Autodesk Inventor part; units mm, degrees
ref_plane "YZ Plane" through (0, 0, 0) normal (1, 0, 0) x (0, 1, 0)
ref_plane "XZ Plane" through (0, 0, 0) normal (0, 1, 0) x (-1, 0, 0)
ref_plane "XY Plane" through (0, 0, 0) normal (0, 0, 1) x (1, 0, 0)
sketch "Sketch1" plane through (0, 0, 0) normal (1, 0, 0) x (0, 1, 0)
  line L0 (-1.5875, -355.6) -> (1.5875, -355.6) construction
  line L1 (1.5875, -355.6) -> (1.5875, 355.6) construction
  line L2 (1.5875, 355.6) -> (-1.5875, 355.6) construction
  line L3 (-1.5875, 355.6) -> (-1.5875, -355.6) construction
  line L4 (-1.5875, -355.6) -> (1.5875, 355.6) construction
  line L5 (1.5875, -355.6) -> (-1.5875, 355.6) construction
  line L6 (52.3875, 152.4) -> (1.5875, 152.4) construction
  line L7 (1.5875, 152.4) -> (1.5875, 127) construction
  line L8 (1.5875, 127) -> (52.3875, 127) construction
  line L9 (52.3875, 127) -> (52.3875, 152.4) construction
  line L10 (52.3875, 152.4) -> (1.5875, 127) construction
  line L11 (1.5875, 152.4) -> (52.3875, 127) construction
  line L12 (77.7875, 177.8) -> (1.5875, 177.8) construction
  line L13 (1.5875, 177.8) -> (1.5875, 152.4) construction
  line L14 (1.5875, 152.4) -> (77.7875, 152.4) construction
  line L15 (77.7875, 152.4) -> (77.7875, 177.8) construction
  line L16 (77.7875, 177.8) -> (1.5875, 152.4) construction
  line L17 (1.5875, 177.8) -> (77.7875, 152.4) construction
  line L18 (900.1125, 152.4) -> (87.3125, 152.4) construction
  line L19 (87.3125, 152.4) -> (87.3125, 177.8) construction
  line L20 (87.3125, 177.8) -> (900.1125, 177.8) construction
  line L21 (900.1125, 177.8) -> (900.1125, 152.4) construction
  line L22 (900.1125, 152.4) -> (87.3125, 177.8) construction
  line L23 (87.3125, 152.4) -> (900.1125, 177.8) construction
  line L24 (87.3125, 177.8) -> (77.7875, 177.8) construction
  line L25 (77.7875, 177.8) -> (77.7875, -177.8) construction
  line L26 (77.7875, -177.8) -> (87.3125, -177.8) construction
  line L27 (87.3125, -177.8) -> (87.3125, 177.8) construction
  line L28 (87.3125, 177.8) -> (77.7875, -177.8) construction
  line L29 (77.7875, 177.8) -> (87.3125, -177.8) construction
  line L30 (82.55, 0) -> (-1.5875, 0) construction
  line L31 (1.5875, -355.6) -> (-1.5875, -355.6) construction
  line L32 (52.3875, -152.4) -> (1.5875, -152.4) construction
  line L33 (1.5875, -152.4) -> (1.5875, -127) construction
  line L34 (1.5875, -127) -> (52.3875, -127) construction
  line L35 (52.3875, -127) -> (52.3875, -152.4) construction
  line L36 (52.3875, -152.4) -> (1.5875, -127) construction
  line L37 (1.5875, -152.4) -> (52.3875, -127) construction
  line L38 (77.7875, -177.8) -> (1.5875, -177.8) construction
  line L39 (1.5875, -177.8) -> (1.5875, -152.4) construction
  line L40 (1.5875, -152.4) -> (77.7875, -152.4) construction
  line L41 (77.7875, -152.4) -> (77.7875, -177.8) construction
  line L42 (77.7875, -177.8) -> (1.5875, -152.4) construction
  line L43 (1.5875, -177.8) -> (77.7875, -152.4) construction
  line L44 (900.1125, -152.4) -> (87.3125, -152.4) construction
  line L45 (87.3125, -152.4) -> (87.3125, -177.8) construction
  line L46 (87.3125, -177.8) -> (900.1125, -177.8) construction
  line L47 (900.1125, -177.8) -> (900.1125, -152.4) construction
  line L48 (900.1125, -152.4) -> (87.3125, -177.8) construction
  line L49 (87.3125, -152.4) -> (900.1125, -177.8) construction
  line L50 (87.3125, -177.8) -> (77.7875, -177.8) construction
  circle A0 centre (66.6623, 160.02) radius 10.3124 construction
  circle A1 centre (66.6623, -160.02) radius 10.3124 construction
  line L51 (138.1125, 176.2125) -> (138.1125, 109.4105) construction
  line L52 (138.1125, 109.4105) -> (-27.5223, 109.4105) construction
  point P0 (0, 0)
  point P1 (26.9875, 139.7)
  point P2 (39.6875, 165.1)
  point P3 (1.5875, 165.1)
  point P4 (493.7125, 165.1)
  point P5 (26.9875, -139.7)
  point P6 (39.6875, -165.1)
  point P7 (1.5875, -165.1)
  point P8 (493.7125, -165.1)
  dimension "d0" = 3.175
  dimension "d1" = 711.2
  dimension "d2" = 50.8
  dimension "d3" = 25.4
  dimension "d4" = 139.7
  dimension "d5" = 76.2
  dimension "d6" = 25.4
  dimension "d7" = 812.8
  dimension "d8" = 25.4
  dimension "d9" = 9.525
  dimension "d10" = 355.6
  dimension "d11" = 20.6248
  dimension "d12" = 11.1252
  dimension "d13" = 7.62
  dimension "d23" = 66.802
  dimension "d24" = 50.8
sketch "Sketch3" plane through (0, 0, 0) normal (1, 0, 0) x (0, 1, 0)
  line L0 (77.7875, -152.4) -> (77.7875, -177.8) construction
  circle A0 centre (66.6623, -160.02) radius 10.3124 construction
  line L1 (1.5875, 355.6) -> (-1.5875, 355.6) construction
  line L2 (1.5875, -355.6) -> (1.5875, 355.6) construction
  line L3 (-1.5875, -355.6) -> (1.5875, 355.6) construction
  line L4 (1.5875, -355.6) -> (-1.5875, 355.6) construction
  line L5 (-1.5875, 355.6) -> (-1.5875, -355.6) construction
  line L6 (87.3125, -177.8) -> (87.3125, 177.8) construction
  line L7 (77.7875, 177.8) -> (77.7875, -177.8) construction
  line L8 (-1.5875, -355.6) -> (1.5875, -355.6) construction
  line L9 (1.5875, -355.6) -> (-1.5875, -355.6) construction
  line L10 (1.5875, 152.4) -> (1.5875, 127) construction
  line L11 (82.55, 0) -> (-1.5875, 0) construction
  line L12 (87.3125, 152.4) -> (87.3125, 177.8) construction
  line L13 (77.7875, -177.8) -> (87.3125, -177.8) construction
  line L14 (1.5875, -127) -> (52.3875, -127) construction
  line L15 (52.3875, 152.4) -> (1.5875, 152.4) construction
  line L16 (52.3875, 152.4) -> (1.5875, 127) construction
  line L17 (1.5875, 127) -> (52.3875, 127) construction
  line L18 (52.3875, 127) -> (52.3875, 152.4) construction
  line L19 (1.5875, 152.4) -> (52.3875, 127) construction
  line L20 (1.5875, 152.4) -> (77.7875, 152.4) construction
  line L21 (1.5875, 177.8) -> (1.5875, 152.4) construction
  line L22 (138.1125, 109.4105) -> (-27.5223, 109.4105) construction
  circle A1 centre (66.6623, 160.02) radius 10.3124 construction
  line L23 (138.1125, 176.2125) -> (138.1125, 109.4105) construction
  line L24 (77.7875, 177.8) -> (1.5875, 152.4) construction
  line L25 (77.7875, 177.8) -> (1.5875, 177.8) construction
  line L26 (77.7875, 152.4) -> (77.7875, 177.8) construction
  line L27 (87.3125, 177.8) -> (77.7875, 177.8) construction
  line L28 (1.5875, 177.8) -> (77.7875, 152.4) construction
  line L29 (900.1125, 152.4) -> (87.3125, 152.4) construction
  line L30 (87.3125, 177.8) -> (900.1125, 177.8) construction
  line L31 (900.1125, 152.4) -> (87.3125, 177.8) construction
  line L32 (87.3125, 152.4) -> (900.1125, 177.8) construction
  line L33 (900.1125, -152.4) -> (87.3125, -177.8) construction
  line L34 (87.3125, -177.8) -> (900.1125, -177.8) construction
  line L35 (900.1125, -152.4) -> (87.3125, -152.4) construction
  line L36 (87.3125, -152.4) -> (900.1125, -177.8) construction
  line L37 (900.1125, 177.8) -> (900.1125, 152.4) construction
  line L38 (900.1125, -177.8) -> (900.1125, -152.4) construction
  line L39 (52.3875, -127) -> (52.3875, -152.4) construction
  line L40 (52.3875, -152.4) -> (1.5875, -127) construction
  line L41 (1.5875, -152.4) -> (1.5875, -127) construction
  line L42 (1.5875, -152.4) -> (52.3875, -127) construction
  line L43 (52.3875, -152.4) -> (1.5875, -152.4) construction
  line L44 (1.5875, -152.4) -> (77.7875, -152.4) construction
  line L45 (1.5875, -177.8) -> (77.7875, -152.4) construction
  line L46 (77.7875, -177.8) -> (1.5875, -177.8) construction
  line L47 (1.5875, -177.8) -> (1.5875, -152.4) construction
  line L48 (77.7875, -177.8) -> (1.5875, -152.4) construction
  line L49 (87.3125, -152.4) -> (87.3125, -177.8) construction
  line L50 (87.3125, -177.8) -> (77.7875, -177.8) construction
  circle A2 centre (39.6875, 64.1731) radius 28.6512 construction
  circle A3 centre (65.0875, 99.0981) radius 10.3124 construction
  line L51 (57.4199, 164.5943) -> (14.0091, 76.8819) construction
  circle A4 centre (39.6875, 64.1731) radius 25.4 construction
  circle A5 centre (49.2125, 27.2829) radius 12.7 construction
  circle A6 centre (49.2125, 27.2829) radius 25.4 construction
  circle A7 centre (39.6875, -3.0046) radius 6.35 construction
  circle A8 centre (39.6875, -3.0046) radius 25.4 construction
  circle A9 centre (39.6875, -3.0046) radius 30.48 construction
  circle A10 centre (65.0875, 99.0981) radius 4.7625 construction
  circle A11 centre (39.6875, 64.1731) radius 14.2875
  circle A12 centre (49.2125, 27.2829) radius 14.2875
  circle A13 centre (9.2075, 45.1231) radius 4.7625 construction
  circle A14 centre (9.2075, 19.7231) radius 4.7625 construction
  line L52 (87.3125, 0) -> (87.3125, 86.6661)
  line L53 (87.3125, 86.6661) -> (68.1488, 102.7464)
  circle A15 centre (42.8625, 99.0981) radius 4.7625 construction
  line L54 (65.0875, 103.8606) -> (42.8625, 103.8606)
  line L55 (38.8212, 101.6179) -> (5.1662, 47.6429)
  line L56 (4.445, 45.1231) -> (4.445, 0)
  arc A16 (68.1488, 102.7464) -> (65.0875, 103.8606) centre (65.0875, 99.0981) ccw
  arc A17 (42.8625, 103.8606) -> (38.8212, 101.6179) centre (42.8625, 99.0981) ccw
  arc A18 (5.1662, 47.6429) -> (4.445, 45.1231) centre (9.2075, 45.1231) ccw
  line L57 (87.3125, 0) -> (87.3125, -86.6661)
  line L58 (87.3125, -86.6661) -> (68.1488, -102.7464)
  line L59 (65.0875, -103.8606) -> (42.8625, -103.8606)
  line L60 (38.8212, -101.6179) -> (5.1662, -47.6429)
  line L61 (4.445, -45.1231) -> (4.445, 0)
  arc A19 (65.0875, -103.8606) -> (68.1488, -102.7464) centre (65.0875, -99.0981) ccw
  arc A20 (38.8212, -101.6179) -> (42.8625, -103.8606) centre (42.8625, -99.0981) ccw
  arc A21 (4.445, -45.1231) -> (5.1662, -47.6429) centre (9.2075, -45.1231) ccw
  circle A22 centre (39.6875, -3.0046) radius 7.62
  circle A23 centre (39.6875, -64.1731) radius 14.2875
  circle A24 centre (49.2125, -27.2829) radius 14.2875
  point P0 (0, 0)
  point P1 (0, 0)
  point P2 (26.9875, 139.7)
  point P3 (1.5875, 165.1)
  point P4 (39.6875, 165.1)
  point P5 (493.7125, -165.1)
  point P6 (493.7125, 165.1)
  point P7 (26.9875, -139.7)
  point P8 (1.5875, -165.1)
  point P9 (39.6875, -165.1)
  point P10 (65.0875, -3.0046)
  point P11 (52.3875, 18.9924)
  point P12 (26.9875, 18.9924)
  point P13 (14.2875, -3.0046)
  point P14 (26.9875, -25.0017)
  point P15 (52.3875, -25.0017)
  point P16 (82.55, 76.2)
  point P17 (82.55, 25.4)
  point P18 (82.55, 177.8)
  dimension "d30" = 57.3024
  dimension "d36" = 50.8
  dimension "d31" = 12.7
  dimension "d32" = 50.8
  dimension "d33" = 25.4
  dimension "d34" = 50.8
  dimension "d35" = 12.7
  dimension "d37" = 60.96
  dimension "d38" = 38.1
  dimension "d39" = 34.925
  dimension "d40" = 9.525
  dimension "d41" = 28.575
  dimension "d42" = 28.575
  dimension "d45" = 360
  dimension "d47" = 50.8
  dimension "d48" = 25.4
  dimension "d49" = 22.225
  dimension "d50" = 7.62
  dimension "d51" = 25.4
  dimension "d52" = 19.05
  dimension "d55" = 130
  dimension "d66" = 15.24
  dimension "d68" = 28.575
  dimension "d69" = 38.1
extrude "Extrusion1" add sketch "Sketch3" along normal blind 6.35
hole "Mount Holes" at (0, 87.3125, -177.8) at (0, 77.7875, -152.4) at (0, 77.7875, -177.8) at (0, 1.5875, 355.6) at (0, -1.5875, 355.6) at (0, 1.5875, 127) at (0, 1.5875, 152.4) at (0, -27.5223, 109.4105) at (0, 0, 0) at (0, 82.55, 0) at (0, 87.3125, 152.4) at (0, 87.3125, 177.8) at (0, 138.1125, 176.2125) at (0, 52.3875, 152.4) at (0, 26.9875, 139.7) at (0, 52.3875, 127) at (0, 1.5875, 165.1) at (0, 39.6875, 165.1) at (0, 77.7875, 152.4) at (0, 66.6623, 160.02) at (0, 493.7125, -165.1) at (0, 493.7125, 165.1) at (0, 26.9875, -139.7) at (0, 66.6623, -160.02) at (0, 1.5875, -165.1) at (0, 39.6875, -165.1) at (0, 52.3875, -25.0017) at (0, 82.55, 76.2) at (0, 82.55, 25.4) at (0, 42.8625, 99.0981) at (0, 9.2075, 45.1231) at (0, 9.2075, 19.7231) direction (1, 0, 0) diameter 5.1054 end through all
hole "Motor Mount" at (0, 77.7875, -177.8) at (0, 65.0875, -3.0046) at (0, 52.3875, 18.9924) at (0, 26.9875, 18.9924) at (0, 14.2875, -3.0046) at (0, 26.9875, -25.0017) direction (1, 0, 0) diameter 5.1054 end through all
mirror "Mirror1" about plane through (0, 0, 0) normal (0, 0, 1) of "Mount Holes"
properties part number "Gearbox sketch" material "Aluminum 6061"
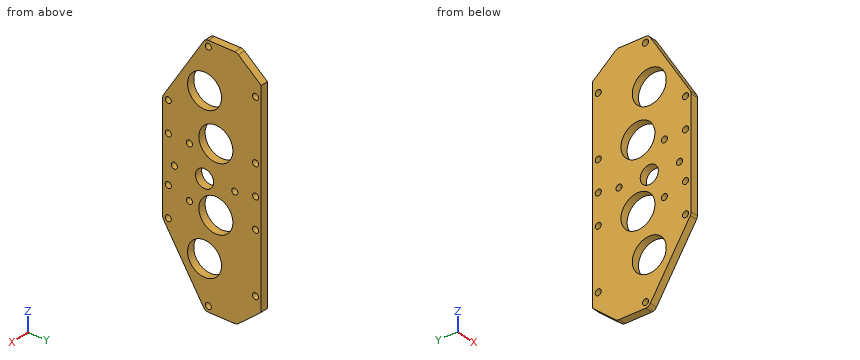
CAD build for the part. Positions are in the model's coordinates, mm. Coordinates: 2 decimals unless noted, no trailing zeros. Loops run counter-clockwise (first coordinate to the right, second up) from the corner with the lowest first, then second, coordinate; pieces in that order, holes last. Notation, with made-up numbers: (70.25, -9.75) - (93.25, -9.75) arc R19 ccw to (93.25, 1.25) - close; hole circle Ø4 at (19.5, -7.5). An arc over 180 degrees is marked (long way). Use one line per item in the form item = value. Start each with the question number.
1) Flat gauge pins, fed straight in: pin 1 (4 mm diameter, centred on y = 9.21, z = -45.12, fed in from +X); pin 2 (3 mm diameter, centred on x = 0.5, z = -64.5, fed in from -Y). Where does each tip first touch, or does it go through?
2) Band-saw the part on C-C (x = 4.75). State how many separate pieces and enclosed holes the cut face has, and give its area (3 significant figures).
3) Band-saw the part on A-A (y = 82.55). Give the cut face in (x, z).
4) Drill centre lines: L1, parallel to Y at x = 2, z = 0 (1 decimal); L2, parallel to Y at x = 4.5, z = -4 (1 decimal); L3, parallel to Z at x = 3, y = 55. Where is each one in solid material? Low to high. Write a range as from..to.
Check values:
q1.pin_1 = through
q1.pin_2 = 14.74
q2.separate_pieces = 1
q2.enclosed_holes = 20
q2.area = 11,800 mm2
q3.outline = (0, -90.66) - (6.35, -90.66) - (6.35, -78.75) - (0, -78.75) - close; (0, -73.65) - (6.35, -73.65) - (6.35, -27.95) - (0, -27.95) - close; (0, -22.85) - (6.35, -22.85) - (6.35, -2.55) - (0, -2.55) - close; (0, 2.55) - (6.35, 2.55) - (6.35, 22.85) - (0, 22.85) - close; (0, 27.95) - (6.35, 27.95) - (6.35, 73.65) - (0, 73.65) - close; (0, 78.75) - (6.35, 78.75) - (6.35, 90.66) - (0, 90.66) - close
q4.L1 = 4.4..32.7, 46.7..80, 85.1..87.3
q4.L2 = 4.4..11.9, 16.6..32.1, 47.2..62.7, 67.4..87.3
q4.L3 = -103.86..-40.35, -14.22..14.22, 40.35..103.86
